Read the model definition and answer for the solid it produces. Units are mm, in the model's axes. A direction names the side the tool comes from. Round coordinates to 2 decimals unless told otherwise and drop trailing zeros. Loops run counter-clockwise (first coordinate to the right, second up) from the corner with the lowest first, then second, coordinate; pieces in that order, holes last. Notation, with made-up numbers: (44.5, -15.75) -> (70.5, -15.75) arc R13 ccw to (70.5, 9.25) -> close; hole circle Ø4 at (-10, 8). An arc over 180 degrees is marked (long way). Put each result on its own line as item: value.
from build123d import *

# Parameters (mm, degrees)
F0_W         = 50
F0_H         = 60
F1_DEPTH     = 1.5
F2_W         = 20
F2_H         = 2
F3_DEPTH     = 9
F4_W         = 6
F4_H         = 5.5
F5_DEPTH     = 32
F6_W         = 44.5
F6_H         = 44.5
F7_DEPTH     = 4.5
F8_R         = 3
F9_T4_DEPTH  = 1.5
F9_T9_DEPTH  = 1.5
F9_T14_DEPTH = 1.5
F9_T19_DEPTH = 1.5


# Not quite as in the source:
# - a fillet or chamfer that OpenCascade refuses, or shapes differently, is made with other operations: its cross-section is extruded or revolved along the edge and cut away or added
# - a feature of the source that left no trace in its solid (it failed there, or was rolled back) is left out


with BuildPart() as f1:
    # F0 (on Top) → F1 (new body)
    with BuildSketch(Plane.XY):
        Rectangle(F0_W, F0_H)
    extrude(amount=F1_DEPTH)

    # F2 (on Top) → F3 (join)
    with BuildSketch(Plane.XY):
        with Locations((10, 31)):
            Rectangle(F2_W, F2_H)
        with Locations((-10, 31)):
            Rectangle(F2_W, F2_H)
        with Locations((-10, -31)):
            Rectangle(F2_W, F2_H)
        with Locations((10, -31)):
            Rectangle(F2_W, F2_H)
    extrude(amount=F3_DEPTH)

    # F4 (on Front) → F5 (cut, symmetric)
    with BuildSketch(Plane.XZ):
        with Locations((-14.75, 4.25)):
            Rectangle(F4_W, F4_H)
        with Locations((14.75, 4.25)):
            Rectangle(F4_W, F4_H)
    extrude(amount=F5_DEPTH, both=True, mode=Mode.SUBTRACT)

    # F6 (on Top) → F7 (join)
    with BuildSketch(Plane.XY):
        Rectangle(F6_W, F6_H)
    extrude(amount=F7_DEPTH)

    # F8
    f8_edges = [f1.edges().sort_by_distance(p)[0] for p in [
        (22.25, -22.25, 3),
        (-22.25, -22.25, 3),
        (-22.25, 22.25, 3),
        (22.25, 22.25, 3),
    ]]
    fillet(f8_edges, radius=F8_R)

    # F9: chamfer of 2 x 5.4949548389 on 4 edges, made by hand


with BuildPart() as f9_tool2:
    # F9_s3 → F9_t4 (new body)
    with BuildSketch(Plane.XY):
        Polygon((25.4949548389, 30), (20, 32), (20, 30), align=None)
    extrude(amount=F9_T4_DEPTH)

    split(bisect_by=Plane.YZ.offset(25), keep=Keep.BOTTOM)


with BuildPart() as f1_1:
    add(f1.part)

    # F9_t1: union F9_tool2
    add(f9_tool2.part)


with BuildPart() as f9_tool7:
    # F9_s8 → F9_t9 (new body)
    with BuildSketch(Plane.XY):
        Polygon((-25.4949548389, -30), (-20, -32), (-20, -30), align=None)
    extrude(amount=F9_T9_DEPTH)

    split(bisect_by=Plane.YZ.offset(-25), keep=Keep.TOP)


with BuildPart() as f1_2:
    add(f1_1.part)

    # F9_t6: union F9_tool7
    add(f9_tool7.part)


with BuildPart() as f9_tool12:
    # F9_s13 → F9_t14 (new body)
    with BuildSketch(Plane.XY):
        Polygon((-25.4949548389, 30), (-20, 32), (-20, 30), align=None)
    extrude(amount=F9_T14_DEPTH)

    split(bisect_by=Plane.YZ.offset(-25), keep=Keep.TOP)


with BuildPart() as f1_3:
    add(f1_2.part)

    # F9_t11: union F9_tool12
    add(f9_tool12.part)


with BuildPart() as f9_tool17:
    # F9_s18 → F9_t19 (new body)
    with BuildSketch(Plane.XY):
        Polygon((25.4949548389, -30), (20, -32), (20, -30), align=None)
    extrude(amount=F9_T19_DEPTH)

    split(bisect_by=Plane.YZ.offset(25), keep=Keep.BOTTOM)


with BuildPart() as f1_4:
    add(f1_3.part)

    # F9_t16: union F9_tool17
    add(f9_tool17.part)


solid = f1_4.part
Item 1: The part is cut by section B-B (z = 8). Determine the outline of the cut face in (x, y).
Derived:
outline: (-20, -32) -> (20, -32) -> (20, -30) -> (-20, -30) -> close; (-20, 30) -> (20, 30) -> (20, 32) -> (-20, 32) -> close
Item 2: The part is cut by section C-C (z = 3). State how many separate pieces and enclosed holes the cut face has, then the cut area to 3 significant figures.
Derived:
separate pieces: 7
enclosed holes: 0
area: 2,080 mm^2
Item 3: Find the intervals of material crossed by line 1 along Y through (x, z) = (-13, 7.75); line 2 along Z through (x, y) = (5, 9.5); line 3 along Z through (x, y) = (20.5, 26.5), in increasing order.
Derived:
line 1: y = -32 to -30, 30 to 32
line 2: z = 0 to 4.5
line 3: z = 0 to 1.5
Item 4: Flat-ended cylindrical pins translate along their axes: pin 1 Ø15 at (x, y) = (-6, -11.5) entering from +Z; pin 2 Ø1 at (x, y) = (16, 31) entering from -Z; pin 3 Ø2.5 at (y, z) = (-6, 3.5) entering from -X; pin 4 Ø2.5 at (y, z) = (-0.5, 3) entering from +X. Find the tip coordinate at first contact, or state that the pin passes through.
Derived:
pin 1: stops at z = 4.5
pin 2: stops at z = 0
pin 3: stops at x = -22.25
pin 4: stops at x = 22.25
Item 5: The part is cut by section A-A (x = 17). Determine the outline of the cut face in (y, z).
Derived:
outline: (-32, 0) -> (32, 0) -> (32, 1.5) -> (22.25, 1.5) -> (22.25, 4.5) -> (-22.25, 4.5) -> (-22.25, 1.5) -> (-32, 1.5) -> close; (-32, 7) -> (-30, 7) -> (-30, 9) -> (-32, 9) -> close; (30, 7) -> (32, 7) -> (32, 9) -> (30, 9) -> close
Item 6: Which of the six approach directions +Z, -Z, +X, -X, +Y, -Y give full straight-line access (tool end or side, diameter ignored) to faces 1 (the flat face through (15, 31, 7)), 2 (the flat face through (-17.75, -31, 4)), 3 (the flat face through (20, -31, 5)), 4 (the flat face through (22.25, 0, 3)), 5 (the flat face through (-17.75, 31, 4))?
Derived:
face 1: +Y, -Y
face 2: -Y
face 3: +Z, +X, -Y
face 4: +Z, +X, +Y, -Y
face 5: +Y
Item 7: The part is cut by section D-D (y = 2.5). Determine the outline of the cut face in (x, z).
Derived:
outline: (-25, 0) -> (25, 0) -> (25, 1.5) -> (22.25, 1.5) -> (22.25, 4.5) -> (-22.25, 4.5) -> (-22.25, 1.5) -> (-25, 1.5) -> close
Item 8: For a pull along Y with two mould halves and no side action, classify faces 6 (the flat face through (0, 30, 5)), 7 (the flat face through (17.75, 31, 4)), 8 (the flat face through (-22.535, 31.077, 0.74)) as pulls with the +Y half, pulls with the -Y half, needs draft (parallel to the pull), parting line crosses it, or undercut.
Derived:
face 6: undercut
face 7: needs draft
face 8: pulls with the +Y half
